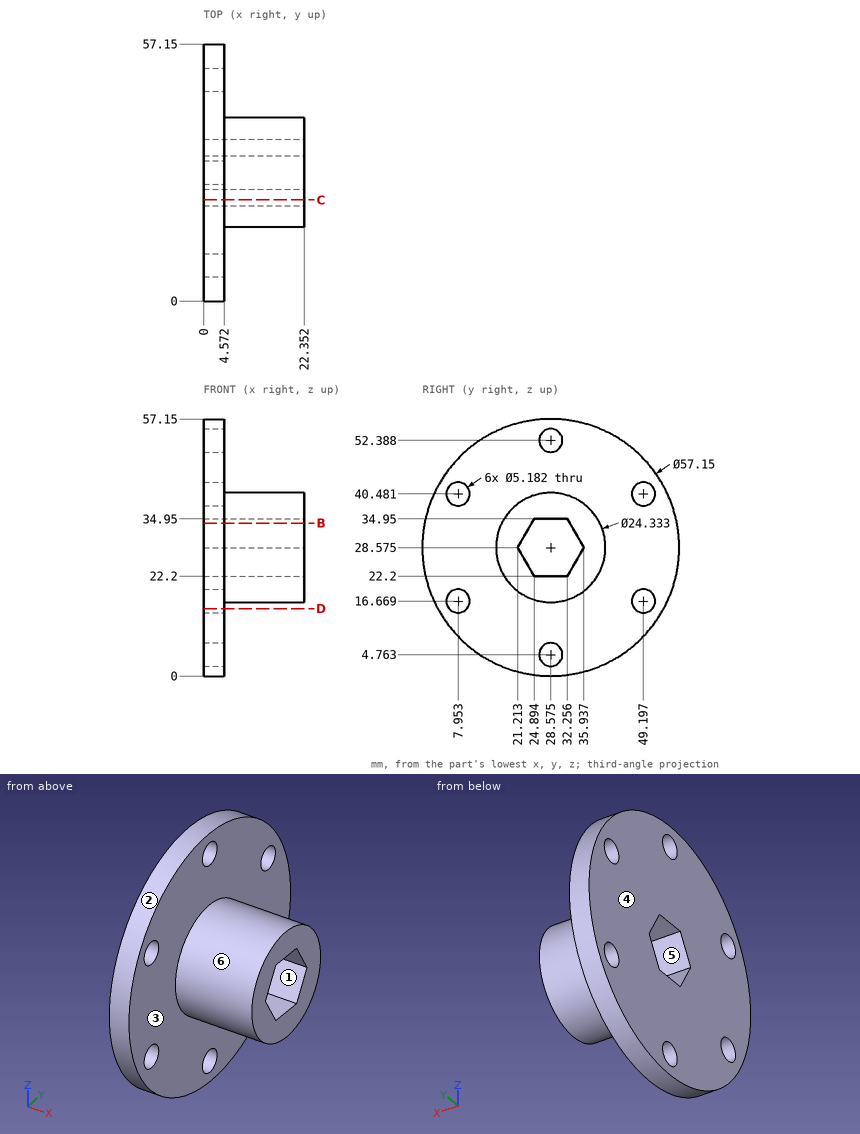
Check sheet for the drawn part. Datum: minimum x, y, z corner. Units: mm. A direction names the side the tool comes from. Round coordinates to 2 decimals unless told otherwise and drop trailing zeros. Loops run counter-clockwise (first coordinate to the right, second up) from the corner with the lowest first, then second, coordinate; pieces in that order, holes last. Notation, with made-up numbers: (64.25, 70) - (74.25, 70) arc R23 cw to (74.25, 106) - close; hole circle Ø4 at (57, 65.5). An arc over 180 degrees is marked (long way). Write each question's results on one line, items separated by ' | '. Start each with the question number.
Q1. Thickness scan on line 1 (Y direction, x = 18.5, z = 28) (1 decimal); line 2 (X direction, y = 37.5, z = 46); line 3 (Z direction, x = 11.25, y = 21.5) (1 decimal). Record the ranges inside material, lowest first. Write a range as [from, to].
Q2. Cross-section at B-B on z = 34. Enter the section's corners in (x, y) (1 decimal).
Q3. Cross-section at D-D on z = 15. Enter the section's corners in (x, y) (1 decimal), and give its area (3 significant figures).
Q4. Gauge pin test, flat ends, axial feed: P1, Ø6, axis at y = 7.95, z = 16.67, coming from the +X side; P2, Ø12, axis at x = 11.5, z = 14.5, coming from the -Y side (1 decimal); P3, Ø4.5, axis at y = 28.58, z = 52.39, coming from the +X side; P4, Ø8, axis at x = 17.5, z = 22.5, coming from the -Y side. Record the tip position at first contact, or that the pin passes through.
Q5. Release check for a two-part mould opening along Y. For the marked faces 1, 2 and 3 record: +Y half, -Y half, draft (parallel to the pull), parting line (faces both ways), or undercut.
Q6. Access from +Z, -Z, +X, -X, +Y, -Y to the whole of each face (thin tool, end or side, straight path). Record for the marked faces 4, 5 and 6.
Q7. Cross-section at C-C on y = 22.5. Enter the section's corners in (x, z).
Answers below:
1) line 1: y = [16.4, 21.5], [35.6, 40.7] | line 2: x = [0, 4.57] | line 3: z = [18.7, 28.1], [29.1, 38.5]
2) outline: (0, 0.5) - (4.6, 0.5) - (4.6, 17.7) - (22.4, 17.7) - (22.4, 24.3) - (0, 24.3) - close; (0, 32.8) - (22.4, 32.8) - (22.4, 39.5) - (4.6, 39.5) - (4.6, 56.6) - (0, 56.6) - close
3) outline: (0, 3.4) - (4.6, 3.4) - (4.6, 6) - (0, 6) - close; (0, 9.9) - (4.6, 9.9) - (4.6, 47.2) - (0, 47.2) - close; (0, 51.2) - (4.6, 51.2) - (4.6, 53.7) - (0, 53.7) - close | area: 194 mm²
4) P1: stops at x = 4.57 | P2: stops at y = 19.5 | P3: passes through | P4: stops at y = 16.59
5) face 1: undercut | face 2: parting line | face 3: draft
6) face 4: +Z, -Z, -X, +Y, -Y | face 5: +X, -X | face 6: +X
7) outline: (0, 0.65) - (4.57, 0.65) - (4.57, 18.03) - (22.35, 18.03) - (22.35, 26.35) - (0, 26.35) - close; (0, 30.8) - (22.35, 30.8) - (22.35, 39.12) - (4.57, 39.12) - (4.57, 56.5) - (0, 56.5) - close
